Answer from the drawing. Dimensions are ordinates in mm from the lowest x, y and z of the part. A direction names the side the tool comes from. Round coordinates to 2 decimals unless told otherwise and drop trailing zeros. Order: outer loops, then holes, each group sorted by start corner. A loop starts at its lowest first (then second) coordinate and runs counter-clockwise, first axis right, second up.
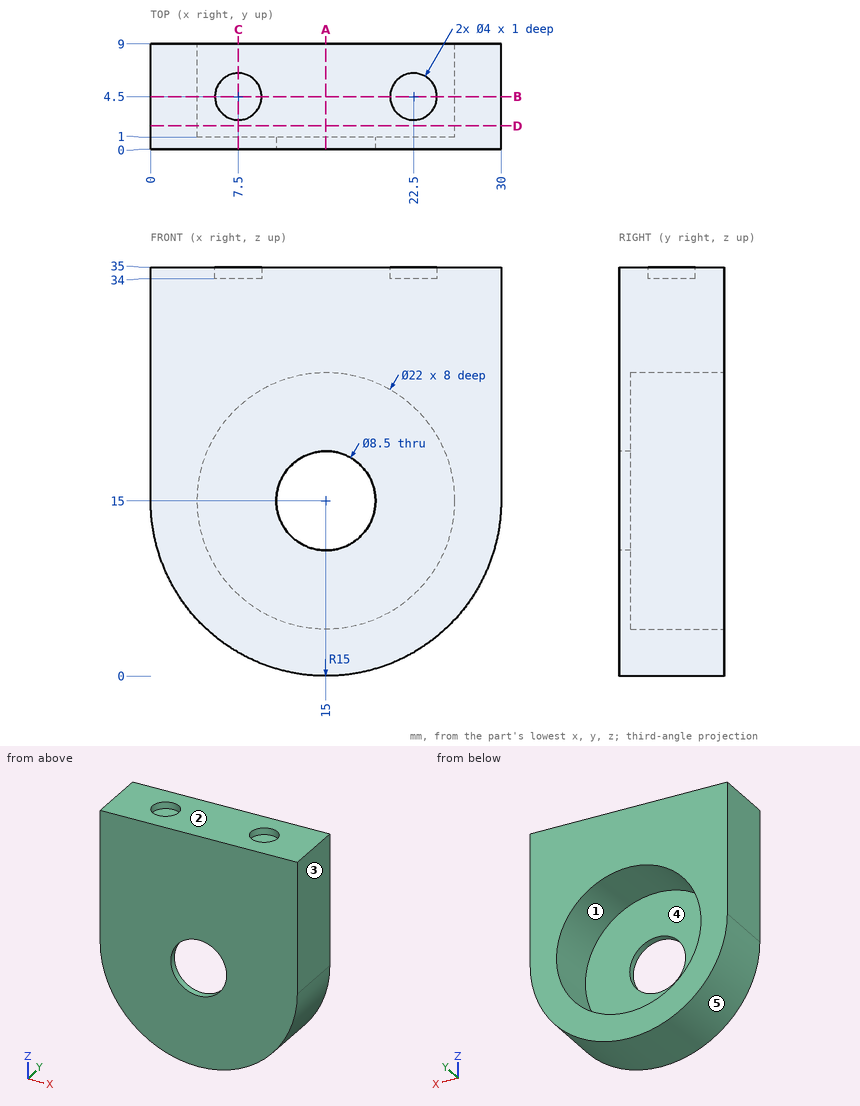
Q1. Straight lines are drawn through the part: probe 1 along Y at (x, z) = (22.5, 34.6); probe 2 along X at (y, z) = (0.3, 15); probe 3 along Z at (x, y) = (15, 0.2). For each, find the intervals that lie inside material, in ascending order.
Outcome:
probe 1: y = 0 to 2.5, 6.5 to 9
probe 2: x = 0 to 10.75, 19.25 to 30
probe 3: z = 0 to 10.75, 19.25 to 35
Q2. A cutting plane is placed at A-A, the plane x = 15. Give the vertices of the cut face in (y, z).
Outcome:
outline: (0, 0) - (9, 0) - (9, 4) - (1, 4) - (1, 10.75) - (0, 10.75) - close; (0, 19.25) - (1, 19.25) - (1, 26) - (9, 26) - (9, 35) - (0, 35) - close
Q3. A cutting plane is placed at D-D, the plane y = 2. Give the vertices of the cut face in (x, z), plus the area to 3 significant figures.
Outcome:
outline: (0, 15) arc R15 ccw to (30, 15) - (30, 35) - (0, 35) - close; hole circle Ø22 at (15, 15)
area: 573 mm2
Q4. A cutting plane is placed at C-C, the plane x = 7.5. Give the vertices of the cut face in (y, z).
Outcome:
outline: (0, 2.01) - (9, 2.01) - (9, 6.95) - (1, 6.95) - (1, 23.05) - (9, 23.05) - (9, 35) - (6.5, 35) - (6.5, 34) - (2.5, 34) - (2.5, 35) - (0, 35) - close
Q5. A cutting plane is placed at B-B, the plane y = 4.5. Give the vertices of the cut face in (x, z), plus the area to 3 significant figures.
Outcome:
outline: (0, 15) arc R15 ccw to (30, 15) - (30, 35) - (24.5, 35) - (24.5, 34) - (20.5, 34) - (20.5, 35) - (9.5, 35) - (9.5, 34) - (5.5, 34) - (5.5, 35) - (0, 35) - close; hole circle Ø22 at (15, 15)
area: 565 mm2
Q6. Flat-ended cylindrical pins translate along their axes: pin 1 (3 mm diameter, centred on x = 6.5, y = 7.5, fed in from -Z); pin 2 (2 mm diameter, centred on x = 7.5, z = 13.5, fed in from +Y); pin 3 (1.2 mm diameter, centred on x = 23, y = 4, fed in from +Z). Find the tip coordinate at first contact, or state that the pin passes through.
Outcome:
pin 1: stops at z = 1.73
pin 2: stops at y = 1
pin 3: stops at z = 34
Q7. For the marked faces 4 and 5, determine the directions among +Z, -Z, +X, -X, +Y, -Y from which every point of the face is accessible in a straight line to the end or side of a thin tool.
Outcome:
face 4: +Y
face 5: -Z, +Y, -Y
Q8. For a pull along Z with two mould halves and no side action, classify the marked faces 1, 2 and 3 as released by +Z, released by -Z, zero draft, split by the parting line, or undercut.
Outcome:
face 1: undercut
face 2: released by +Z
face 3: zero draft
